Could you check a few things on this model? Use its own coordinates, in mm. Face numbers are marked on the shaded views. A direction names the side the tool comes from. Coordinates: 2 decimals unless noted, no trailing zeros. Write each loop counter-clockwise with the first axis right and the second up, starting at its lowest first coordinate (ties: lowest second). Pieces come first, ordered by that corner, then holes.
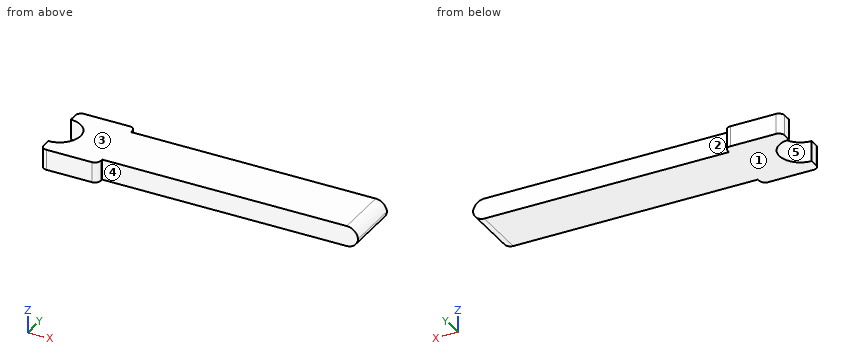
```python
from build123d import *

# Parameters (mm, degrees)
F1_DEPTH    = 9.144
F2_R        = 2.54
F3_W        = 24.13
F3_H        = 9.144
F4_DEPTH    = 114.3
F5_T1_DEPTH = 49.53


# Not quite as in the source:
# - a fillet or chamfer that OpenCascade refuses, or shapes differently, is made with other operations: its cross-section is extruded or revolved along the edge and cut away or added


with BuildPart() as f1:
    # F0 (on Top) → F1 (new body)
    with BuildSketch(Plane.XY):
        with BuildLine():
            ThreePointArc((0, 9.398), (9.398, 0), (0, -9.398))
            Line((0, -9.398), (0, -15.748))
            Line((0, -15.748), (25.4, -15.748))
            Line((25.4, -15.748), (25.4, 15.748))
            Line((25.4, 15.748), (0, 15.748))
            Line((0, 15.748), (0, 9.398))
        make_face()
    extrude(amount=F1_DEPTH)

    # F2
    f2_edges = [f1.edges().sort_by_distance(p)[0] for p in [
        (25.4, -15.748, 4.572),
        (0, -15.748, 4.572),
        (0, 15.748, 4.572),
        (25.4, 15.748, 4.572),
    ]]
    fillet(f2_edges, radius=F2_R)

    # F3 (on face) → F4 (join)
    with BuildSketch(Plane.YZ.offset(25.4)):
        with Locations((0, 4.572)):
            Rectangle(F3_W, F3_H)
    extrude(amount=F4_DEPTH)

    # F5: fillet of radius 5.08 on 2 edges, made by hand

    # F5_s2 → F5_t1 (cut)
    with BuildSketch(Plane.XZ.offset(-24.765)):
        with BuildLine():
            ThreePointArc((134.62, 9.144), (138.2121024484, 7.6561024484), (139.7, 4.064))
            Line((139.7, 4.064), (139.7, 9.144))
            Line((139.7, 9.144), (134.62, 9.144))
        make_face()
        with BuildLine():
            ThreePointArc((134.62, 0), (138.2121024484, 1.4878975516), (139.7, 5.08))
            Line((139.7, 5.08), (139.7, 0))
            Line((139.7, 0), (134.62, 0))
        make_face()
    extrude(amount=F5_T1_DEPTH, mode=Mode.SUBTRACT)


solid = f1.part
```
Item 1: I want a section at C-C, the plane z = 6.25. List the corners of the cut face in (x, y) for me (3 decimals).
Item 2: Will these pins go through, and if not, where does the flat tip stop? pin 1 Ø1.3 at (y, z) = (-13, 6.5) entering from +X; pin 2 Ø4 at (y, z) = (-7, 7.5) entering from +X; pin 3 Ø2.5 at (x, z) = (90.5, 2.5) entering from -Y (3 decimals).
Item 3: If I drill on line 1 along Y through (x, z) = (81.5, 4.75) (3 decimals); line 2 along Y through (x, z) = (7, 7.75); line 3 along X through (y, z) = (3, 5), over which ranges is the centre line in solid material (lowest first)?
Item 4: If we mould it in two halves opening along Y, with no side actions, what happens to the marked faces 3, 4 and 5? For each: released by +Y, released by -Y, zero draft, split by the parting line, or undercut.
Item 5: I want a section at B-B, the plane x = 8. List the corners of the cut face in (y, z) for me.
Item 6: Which directions (+Z, -Z, +X, -X, +Y, -Y) give clear straight access to the entire face, cutting with the end or side of a thin tool? Please do the marked faces 1 and 2.
Item 7: I want a section at A-A, the plane y = 0. List the corners of the cut face in (x, z) for me.
Item 8: I want a section at D-D, the plane x = 92.5. List the corners of the cut face in (y, z) for me (3 decimals), then the cut area to 3 significant figures.
Taken from the geometry:
1. outline: (0, -13.208) arc R2.54 ccw to (2.54, -15.748) - (22.86, -15.748) arc R2.54 ccw to (25.4, -13.208) - (25.4, -12.065) - (139.206, -12.065) - (139.206, 12.065) - (25.4, 12.065) - (25.4, 13.208) arc R2.54 ccw to (22.86, 15.748) - (2.54, 15.748) arc R2.54 ccw to (0, 13.208) - (0, 9.398) arc R9.398 cw to (0, -9.398) - close
2. pin 1: stops at x = 25.4
2. pin 2: stops at x = 139.49
2. pin 3: stops at y = -12.065
3. line 1: y = -12.065 to 12.065
3. line 2: y = -15.75 to -6.27, 6.27 to 15.75
3. line 3: x = 8.91 to 139.61
4. face 3: zero draft
4. face 4: released by -Y
4. face 5: undercut
5. outline: (-15.75, 0) - (-4.93, 0) - (-4.93, 9.14) - (-15.75, 9.14) - close; (4.93, 0) - (15.75, 0) - (15.75, 9.14) - (4.93, 9.14) - close
6. face 1: -Z, +X, -X, +Y, -Y
6. face 2: +Z, -Z, +X, +Y
7. outline: (9.4, 0) - (134.62, 0) arc R5.08 ccw to (139.67, 4.57) arc R5.08 ccw to (134.62, 9.14) - (9.4, 9.14) - close
8. outline: (-12.065, 0) - (12.065, 0) - (12.065, 9.144) - (-12.065, 9.144) - close
8. area: 221 mm2
